Part model, mm, in its own coordinate system. Face numbers are marked on the shaded views. A direction names the side the tool comes from. Give positions to 0.01 mm unless a question says otherwise; leave off trailing zeros. Order: outer loops, then holes, each group sorted by start corner. A loop starts at its lowest first (then second) coordinate and runs counter-clockwise, first axis right, second up.
1. Slice it at B-B on y = 8. List the corners of the cut face in (x, z).
2. Slice it at A-A on x = 0. List the corners of the cut face in (y, z).
3. Probe line 1 (Z direction, x = -7, y = -4.25); line 2 (Z direction, x = -7, y = -0.25); line 3 (X direction, y = -6.75, z = 1.25). List the from-to ranges inside material, lowest first.
4. Which spindle directions (+Z, -Z, +X, -X, +Y, -Y) get a long thin tool onto all of the face, cutting with end or side? Do the marked faces 1 and 2. Say none if no direction does.
5. Drop flat-ended pins along their axis: pin 1 Ø2 at (y, z) = (5.5, 6.5) entering from +X; pin 2 Ø2 at (x, z) = (-2, 1.5) entering from -Y; pin 3 Ø4 at (y, z) = (-1, 5.5) entering from +X. Give the stop position or say it passes through.
6. Slice it at D-D on y = -4. List the corners of the cut face in (x, z).
7. Slice it at C-C on z = 0.5. List the corners of the cut face in (x, y), and give its area (3 significant figures).
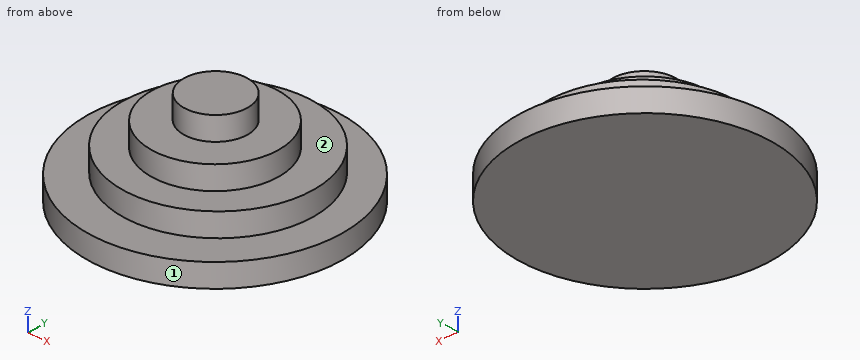
from build123d import *

# Parameters (mm, degrees)
F0_R     = 11
F1_DEPTH = 2
F2_R     = 8.25
F3_DEPTH = 2
F4_R     = 5.5
F5_DEPTH = 2
F6_R     = 2.75
F7_DEPTH = 2


# Not quite as in the source:
# - a feature names something its author has since deleted; it is built from what else it names


with BuildPart() as f1:
    # F0 (on Top) → F1 (new body)
    with BuildSketch(Plane.XY):
        Circle(F0_R)
    extrude(amount=F1_DEPTH)

    # F2 (on face) → F3 (join)
    with BuildSketch(Plane.XY.offset(2)):
        with Locations((0, 0.2906154259)):
            Circle(F2_R)
    extrude(amount=F3_DEPTH)

    # F4 (on face) → F5 (join)
    with BuildSketch(Plane.XY.offset(4)):
        Circle(F4_R)
    extrude(amount=F5_DEPTH)

    # F6 (on face) → F7 (join)
    with BuildSketch(Plane.XY.offset(6)):
        with Locations((0, 0.0671765927)):
            Circle(F6_R)
    extrude(amount=F7_DEPTH)


solid = f1.part
Data:
1. outline: (-7.55, 0) - (7.55, 0) - (7.55, 2) - (2.94, 2) - (2.94, 4) - (-2.94, 4) - (-2.94, 2) - (-7.55, 2) - close
2. outline: (-11, 0) - (11, 0) - (11, 2) - (8.54, 2) - (8.54, 4) - (5.5, 4) - (5.5, 6) - (2.82, 6) - (2.82, 8) - (-2.68, 8) - (-2.68, 6) - (-5.5, 6) - (-5.5, 4) - (-7.96, 4) - (-7.96, 2) - (-11, 2) - close
3. line 1: z = 0 to 2
3. line 2: z = 0 to 4
3. line 3: x = -8.69 to 8.69
4. face 1: +Z, -Z
4. face 2: +Z
5. pin 1: stops at x = 2.96
5. pin 2: stops at y = -10.95
5. pin 3: stops at x = 8.25
6. outline: (-10.25, 0) - (10.25, 0) - (10.25, 2) - (7.05, 2) - (7.05, 4) - (3.77, 4) - (3.77, 6) - (-3.77, 6) - (-3.77, 4) - (-7.05, 4) - (-7.05, 2) - (-10.25, 2) - close
7. outline: circle Ø22 at (0, 0)
7. area: 380 mm2
